Check sheet for the modelled part. Datum: model origin and axes. Units: mm. Face numbers are marked on the shaded views. Coordinates: 2 decimals unless noted, no trailing zeros. Write each loop counter-clockwise with the first axis right and the second up, starting at its lowest first coordinate (ties: lowest second). Pieces come first, ordered by that corner, then holes. Notation, with made-up numbers: (26.5, 38) - (78.5, 38) arc R9 ccw to (78.5, 47) - close; hole circle Ø6 at (63.25, -38). An arc over 180 degrees is marked (long way). Answer as CSV lines item,"result". Start each with the question number.
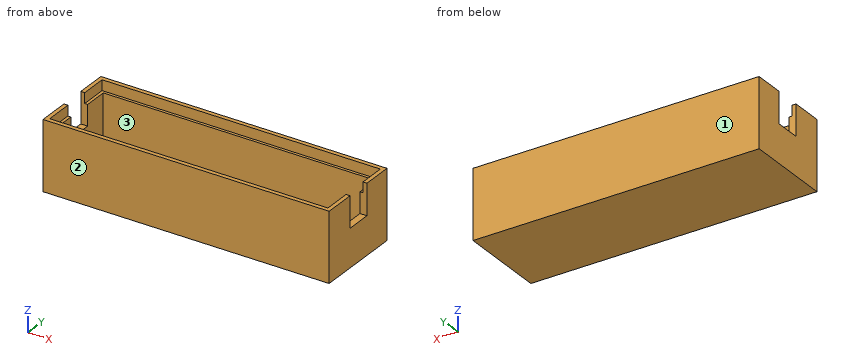
from build123d import *

# Parameters (mm, degrees)
F0_W     = 41.3636378944
F0_H     = 12.7272736281
F1_DEPTH = 10
F2_T     = -1
F3_W     = 40.2219519019
F3_H     = 11.5317674354
F4_DEPTH = 1.5
F5_W     = 3.7121215137
F5_H     = 4.5032251999
F6_DEPTH = 60


with BuildPart() as f1:
    # F0 (on Top) → F1 (new body)
    with BuildSketch(Plane.XY):
        Rectangle(F0_W, F0_H)
    extrude(amount=F1_DEPTH)

    # F2
    f2_openings = [f1.faces().sort_by_distance(p)[0] for p in [
        (0, 0, 10),
    ]]
    offset(amount=F2_T, openings=f2_openings)

    # F3 (on face) → F4 (cut)
    with BuildSketch(Plane.XY.offset(10)):
        Rectangle(F3_W, F3_H)
    extrude(amount=-F4_DEPTH, mode=Mode.SUBTRACT)

    # F5 (on face) → F6 (cut)
    with BuildSketch(Plane(origin=(-20.6818189472, 0, 0), x_dir=(0, -1, 0), z_dir=(-1, 0, 0))):
        with Locations((-0.0884092296, 7.7483874001)):
            Rectangle(F5_W, F5_H)
    extrude(amount=-F6_DEPTH, mode=Mode.SUBTRACT)


solid = f1.part
(1) Material ranges on probe 1 along Y at (x, z) = (5, 1.25); probe 2 along X at (y, z) = (4.5, 5); probe 3 along Y at (x, z) = (-7, 9), recorded low to high. Write a range as from..to.
(2) Go/stop test with flat-tipped pins: P1, Ø1.1, axis at x = 20, y = 0.5, coming from the +Z side; P2, Ø1, axis at x = -4.5, y = -2.5, coming from the +Z side. Record where each tip stops, or that it passes through.
(3) Cross-section at C-C on y = -4. Record the boundary of the cut face in (x, z), plus the area to 3 significant figures.
(4) Cross-section at D-D on x = -4. Record the boundary of the cut face in (y, z), plus the area to 3 significant figures.
(5) Cross-section at B-B on z = 9.5. Record the boundary of the cut face in (x, y), plus the area to 3 significant figures.
(6) Release check for a two-part mould opening along Y. For the marked faces 1, 2 and 3 record: pulls with the +Y half, pulls with the -Y half, needs draft (parallel to the pull), parting line crosses it, or undercut.
(7) Cross-section at A-A on z = 2.5. Record the boundary of the cut face in (x, y).
Checked values:
1,probe 1,"-6.36..-5.36, 5.36..6.36"
1,probe 2,"-20.68..-19.68, 19.68..20.68"
1,probe 3,"-6.36..-5.77, 5.77..6.36"
2,P1,"z = 5.5"
2,P2,"z = 1"
3,outline,"(-20.68, 0) - (20.68, 0) - (20.68, 10) - (20.11, 10) - (20.11, 8.5) - (19.68, 8.5) - (19.68, 1) - (-19.68, 1) - (-19.68, 8.5) - (-20.11, 8.5) - (-20.11, 10) - (-20.68, 10) - close"
3,area,"58.1 mm^2"
4,outline,"(-6.36, 0) - (6.36, 0) - (6.36, 10) - (5.77, 10) - (5.77, 8.5) - (5.36, 8.5) - (5.36, 1) - (-5.36, 1) - (-5.36, 8.5) - (-5.77, 8.5) - (-5.77, 10) - (-6.36, 10) - close"
4,area,"29.5 mm^2"
5,outline,"(-20.68, -6.36) - (20.68, -6.36) - (20.68, -1.77) - (20.11, -1.77) - (20.11, -5.77) - (-20.11, -5.77) - (-20.11, -1.77) - (-20.68, -1.77) - close; (-20.68, 1.94) - (-20.11, 1.94) - (-20.11, 5.77) - (20.11, 5.77) - (20.11, 1.94) - (20.68, 1.94) - (20.68, 6.36) - (-20.68, 6.36) - close"
5,area,"58.4 mm^2"
6,face 1,"pulls with the +Y half"
6,face 2,"pulls with the -Y half"
6,face 3,"undercut"
7,outline,"(-20.68, -6.36) - (20.68, -6.36) - (20.68, 6.36) - (-20.68, 6.36) - close; hole (-19.68, -5.36) - (19.68, -5.36) - (19.68, 5.36) - (-19.68, 5.36) - close"
